Part model, mm, in its own coordinate system. A direction names the side the tool comes from. Coordinates: 2 decimals unless noted, no trailing zeros. Loops run counter-clockwise (first coordinate to the right, second up) from the corner with the lowest first, then second, coordinate; pieces in that order, holes last. Notation, with made-up numbers: (70, 24.25) - (86, 24.25) arc R6 ccw to (86, 29.25) - close; hole circle Ø6 at (-14, 89). An arc over 180 degrees is marked (long way). Use a Markdown table: item, result. Add a question column.
1. Wall check: probe 1 along Y at (x, z) = (2.2, -39); probe 2 along Y at (x, z) = (2.7, -33.5); probe 3 along Y at (x, z) = (2.5, -25). Give the ranges that are in metal, low to high. Write a range as [from, to].
2. 3-axis set-ups, long thin cutter, end or side, ignore diameter. For faces 4 (the flat face through (2, 33.274, -39)), 5 (the flat face through (3.175, 34.4, -26.7)): which of +Z, -Z, +X, -X, +Y, -Y reach the whole face in a straight line?
3. Drop a flat-ended pin along its axis: pin 1 (5.5 mm diameter, centred on y = 34.925, z = -57.15, fed in from +X). Give the stop position or say it passes through.
4. Band-saw the part on C-C, the plane x = 1.1. Give the cut face in (y, z) (3 decimals), plus the area to 3 significant figures.
5. Band-saw the part on A-A, the plane z = -49. Give the cut face in (x, y) (3 decimals).
6. Band-saw the part on B-B, the plane y = 42. Give the cut face in (x, z) (3 decimals).
7. Band-saw the part on D-D, the plane z = -57.15. Give the cut face in (x, y) (3 decimals), plus the area to 3 significant figures.
8. Pull direction Z, two halves, no side cores. Call faces 1 (the flat face through (2, 34, 0)), 2 (the flat face through (0, 34.4, -26.7)), 3 (the flat face through (2, 42.926, -44)): pulls with the +Z half, pulls with the -Z half, needs draft (parallel to the pull), parting line crosses it, or undercut.
from build123d import *

# Parameters (mm, degrees)
F0_W     = 69.85
F0_H     = 69.85
F0_W_2   = 3.302
F0_H_2   = 29.21
F0_R     = 3.332443
F0_H_3   = 15.24
F0_H_4   = 24.13
F1_DEPTH = 3.175


with BuildPart() as f1:
    # F0 (on Right) → F1 (new body)
    with BuildSketch(Plane.YZ):
        with Locations((34.925, -34.925)):
            Rectangle(F0_W, F0_H)
        with Locations((28.575, -36.672557)):
            Rectangle(F0_W_2, F0_H_2, mode=Mode.SUBTRACT)
        with Locations((34.925, -57.15)):
            Circle(F0_R, mode=Mode.SUBTRACT)
        with Locations((41.275, -43.657557)):
            Rectangle(F0_W_2, F0_H_3, mode=Mode.SUBTRACT)
        with Locations((34.925, -39.212557)):
            Rectangle(F0_W_2, F0_H_4, mode=Mode.SUBTRACT)
    extrude(amount=F1_DEPTH)


solid = f1.part
Geometry check:
| question | item | result |
|---|---|---|
| 1 | probe 1 | y = [0, 26.92], [30.23, 33.27], [36.58, 39.62], [42.93, 69.85] |
| 1 | probe 2 | y = [0, 26.92], [30.23, 33.27], [36.58, 69.85] |
| 1 | probe 3 | y = [0, 26.92], [30.23, 69.85] |
| 2 | face 4 | +X, -X |
| 2 | face 5 | +Z, -Z, +X, +Y, -Y |
| 3 | pin 1 | passes through |
| 4 | outline | (0, -69.85) - (69.85, -69.85) - (69.85, 0) - (0, 0) - close; hole (26.924, -51.278) - (30.226, -51.278) - (30.226, -22.068) - (26.924, -22.068) - close; hole circle Ø6.665 at (34.925, -57.15); hole (33.274, -51.278) - (36.576, -51.278) - (36.576, -27.148) - (33.274, -27.148) - close; hole (39.624, -51.278) - (42.926, -51.278) - (42.926, -36.038) - (39.624, -36.038) - close |
| 4 | area | 4,620 mm^2 |
| 5 | outline | (0, 0) - (3.175, 0) - (3.175, 26.924) - (0, 26.924) - close; (0, 30.226) - (3.175, 30.226) - (3.175, 33.274) - (0, 33.274) - close; (0, 36.576) - (3.175, 36.576) - (3.175, 39.624) - (0, 39.624) - close; (0, 42.926) - (3.175, 42.926) - (3.175, 69.85) - (0, 69.85) - close |
| 6 | outline | (0, -69.85) - (3.175, -69.85) - (3.175, -51.278) - (0, -51.278) - close; (0, -36.038) - (3.175, -36.038) - (3.175, 0) - (0, 0) - close |
| 7 | outline | (0, 0) - (3.175, 0) - (3.175, 31.593) - (0, 31.593) - close; (0, 38.257) - (3.175, 38.257) - (3.175, 69.85) - (0, 69.85) - close |
| 7 | area | 201 mm^2 |
| 8 | face 1 | pulls with the +Z half |
| 8 | face 2 | needs draft |
| 8 | face 3 | undercut |
